```python
from build123d import *

# Parameters (mm, degrees)
SCHIZZO1_R                   = 15
SCHIZZO1_R_2                 = 5
ESTRUSIONE_ESTRUSIONE3_DEPTH = 10
ESTRUSIONE_ESTRUSIONE4_DEPTH = 6
RACCORDO1_R                  = 2
RACCORDO2_R                  = 4


with BuildPart() as part:
    # Schizzo1 → Estrusione-Estrusione3 (new, symmetric)
    with BuildSketch(Plane(origin=(0, 0, 0), x_dir=(1, 0, 0), z_dir=(0, 1, 0))):
        with BuildLine():
            Line((-9.947570822, 81.022660617), (-15.953490717, 22.602190996))
            ThreePointArc((-15.953490717, 22.602190996), (-19.887097519, 10.546739253), (-28.450004541, 1.193461616))
            Line((-28.450004541, 1.193461616), (-75.064098517, -31.841096257))
            ThreePointArc((-75.064098517, -31.841096257), (-77.965975808, -44.958742299), (-65.193896965, -49.126179346))
            Line((-65.193896965, -49.126179346), (-11.597326225, -25.117223738))
            ThreePointArc((-11.597326225, -25.117223738), (0.80980464, -22.496101285), (13.191434192, -25.235157478))
            Line((13.191434192, -25.235157478), (65.107247501, -49.0868681))
            ThreePointArc((65.107247501, -49.0868681), (77.918400858, -45.041144531), (75.141467788, -31.896481271))
            Line((75.141467788, -31.896481271), (27.550816942, 2.515032742))
            ThreePointArc((27.550816942, 2.515032742), (19.077292879, 11.949362033), (15.258570349, 24.041695862))
            Line((15.258570349, 24.041695862), (9.956851016, 80.927964356))
            ThreePointArc((9.956851016, 80.927964356), (0.047574951, 89.999886831), (-9.947570822, 81.022660617))
        make_face()
        with Locations(Location((0, 0, 0), (0, 0, 270))):
            Circle(SCHIZZO1_R, mode=Mode.SUBTRACT)
        with Locations(Location((0, 80, 0), (0, 0, 270))):
            Circle(SCHIZZO1_R_2, mode=Mode.SUBTRACT)
        with Locations(Location((69.282032303, -40, 0), (0, 0, 270))):
            Circle(SCHIZZO1_R_2, mode=Mode.SUBTRACT)
        with Locations(Location((-69.282032303, -40, 0), (0, 0, 270))):
            Circle(SCHIZZO1_R_2, mode=Mode.SUBTRACT)
        with BuildLine():
            Line((-5.859435485, 71.896481271), (-11.573917762, 16.31086839))
            ThreePointArc((-11.573917762, 16.31086839), (0, 20), (11.573917762, 16.31086839))
            Line((11.573917762, 16.31086839), (5.859435485, 71.896481271))
            ThreePointArc((5.859435485, 71.896481271), (0, 70), (-5.859435485, 71.896481271))
        make_face(mode=Mode.SUBTRACT)
        with BuildLine():
            Line((65.193896965, -30.873820654), (19.912585265, 1.867872608))
            ThreePointArc((19.912585265, 1.867872608), (17.320508076, -10), (8.338667503, -18.178740998))
            Line((8.338667503, -18.178740998), (59.334461481, -41.022660617))
            ThreePointArc((59.334461481, -41.022660617), (60.621778265, -35), (65.193896965, -30.873820654))
        make_face(mode=Mode.SUBTRACT)
        with BuildLine():
            Line((-59.334461481, -41.022660617), (-8.338667503, -18.178740998))
            ThreePointArc((-8.338667503, -18.178740998), (-17.320508076, -10), (-19.912585265, 1.867872608))
            Line((-19.912585265, 1.867872608), (-65.193896965, -30.873820654))
            ThreePointArc((-65.193896965, -30.873820654), (-60.621778265, -35), (-59.334461481, -41.022660617))
        make_face(mode=Mode.SUBTRACT)
    extrude(amount=ESTRUSIONE_ESTRUSIONE3_DEPTH, both=True)

    # Schizzo1_2 → Estrusione-Estrusione4 (add, symmetric)
    with BuildSketch(Plane(origin=(0, 0, 0), x_dir=(1, 0, 0), z_dir=(0, 1, 0))):
        with BuildLine():
            ThreePointArc((-19.912585265, 1.867872608), (-17.320508076, -10), (-8.338667503, -18.178740998))
            Line((-8.338667503, -18.178740998), (-59.334461481, -41.022660617))
            ThreePointArc((-59.334461481, -41.022660617), (-60.621778265, -35), (-65.193896965, -30.873820654))
            Line((-65.193896965, -30.873820654), (-19.912585265, 1.867872608))
        make_face()
        with BuildLine():
            ThreePointArc((11.573917762, 16.31086839), (0, 20), (-11.573917762, 16.31086839))
            Line((-11.573917762, 16.31086839), (-5.859435485, 71.896481271))
            ThreePointArc((-5.859435485, 71.896481271), (0, 70), (5.859435485, 71.896481271))
            Line((5.859435485, 71.896481271), (11.573917762, 16.31086839))
        make_face()
        with BuildLine():
            ThreePointArc((65.193896965, -30.873820654), (60.621778265, -35), (59.334461481, -41.022660617))
            Line((59.334461481, -41.022660617), (8.338667503, -18.178740998))
            ThreePointArc((8.338667503, -18.178740998), (17.320508076, -10), (19.912585265, 1.867872608))
            Line((19.912585265, 1.867872608), (65.193896965, -30.873820654))
        make_face()
    extrude(amount=ESTRUSIONE_ESTRUSIONE4_DEPTH, both=True)

    # Raccordo1
    raccordo1_edges = [part.edges().sort_by_distance(p)[0] for p in [
        (-59.334461481, -8, 41.022660617),
        (5.859435485, -8, -71.896481271),
        (-5.859435485, -8, -71.896481271),
        (59.334461481, -8, 41.022660617),
        (65.193896965, -8, 30.873820654),
        (5.859435485, 8, -71.896481271),
        (-5.859435485, 8, -71.896481271),
        (59.334461481, 8, 41.022660617),
        (65.193896965, 8, 30.873820654),
        (-65.193896965, 8, 30.873820654),
        (-59.334461481, 8, 41.022660617),
        (-65.193896965, -8, 30.873820654),
    ]]
    fillet(raccordo1_edges, radius=RACCORDO1_R)

    # Raccordo2
    raccordo2_edges = [part.edges().sort_by_distance(p)[0] for p in [
        (11.573917762, -8, -16.31086839),
        (-11.573917762, -8, -16.31086839),
        (8.338667503, -8, 18.178740998),
        (19.912585265, -8, -1.867872608),
        (-11.573917762, 8, -16.31086839),
        (11.573917762, 8, -16.31086839),
        (19.912585265, 8, -1.867872608),
        (8.338667503, 8, 18.178740998),
        (-8.338667503, 8, 18.178740998),
        (-19.912585265, 8, -1.867872608),
        (-19.912585265, -8, -1.867872608),
        (-8.338667503, -8, 18.178740998),
    ]]
    fillet(raccordo2_edges, radius=RACCORDO2_R)


solid = part.part
```
Source: CAD feature listing. Evaluate the final solid. Frame: model axes, mm. A direction names the side the tool comes from. Round coordinates to 2 decimals unless told otherwise and drop trailing zeros. Loops run counter-clockwise (first coordinate to the right, second up) from the corner with the lowest first, then second, coordinate; pieces in that order, holes last. Notation, with made-up numbers: M 55.25,14.5 L 82.25,14.5 A25 ccw 82.25,45.5 Z; hole C -31.75,56.25 d4. An arc over 180 degrees is marked long. Use a Markdown table: item, result. Add a question column.
1. Cut plane D-D, the plane y = 2.5. Output: boundary loops of the cut face in (x, z).
2. Cut plane B-B, the plane z = -10. Output: boundary loops of the cut face in (x, y).
3. Contact query for flat-ended pins moving along their axis: pin 1 (6 mm diameter, centred on x = -31.5, y = -4, fed in from +Z); pin 2 (11.5 mm diameter, centred on x = 69.28, z = 40, fed in from -Y); pin 3 (11.5 mm diameter, centred on x = 29.5, z = 16.5, fed in from -Y); pin 4 (5 mm diameter, centred on x = 22, y = 8, fed in from -Z). Output: stop coordinate, or through.
4. Cut plane C-C, the plane x = -33. Output: boundary loops of the cut face in (y, z), and give its area (3 significant figures).
5. Cut plane A-A, the plane x = 0. Output: boundary loops of the cut face in (y, z), and give its area (3 significant figures).
6. Set-up query: faces 4 (the cylindrical face through (0, 8, -70)), 5 (the flat face through (38, -6, 21)), 6 (the flat face through (38.8, 0.1, 37)). Return all of +Z, -Z, +X, -X, +Y, -Y with unobstructed straight access to the full face (end or side cutting, diameter ignored); none if empty.
7. Ray query, line 1 along X through (y, z) = (8, 27); line 2 along X through (y, z) = (8, 36.5); line 3 along X through (y, z) = (-2, 40). Return the intervals inside material, ascending. Write a range as [from, to].
8. Pull-direction query (X, two-part tool) for faces 1 (the cylindrical face through (-60.647, 7.972, 34.957)), 2 (the flat face through (51.68, 0.14, 14.93)), 3 (the cylindrical face through (-19.8, 0.1, -10.7)); classes: +X half, -X half, draft (parallel to the pull), parting line (faces both ways), or undercut.
Solution:
| question | item | result |
|---|---|---|
| 1 | outline | M -75.06,31.84 L -28.45,-1.19 A30 cw -15.95,-22.6 L -9.95,-81.02 A10 ccw 9.96,-80.93 L 15.26,-24.04 A30 cw 27.55,-2.52 L 75.14,31.9 A10 ccw 65.11,49.09 L 13.19,25.24 A30 cw -11.6,25.12 L -65.19,49.13 A10 ccw Z; hole C -69.28,40 d10; hole C 0,0 d30; hole C 0,-80 d10; hole C 69.28,40 d10 |
| 2 | outline | M -20.21,-10 L -11.18,-10 L -11.18,10 L -20.21,10 Z; M 11.18,-10 L 20.29,-10 L 20.29,10 L 11.18,10 Z |
| 3 | pin 1 | stops at z = 35.38 |
| 3 | pin 2 | stops at y = -10 |
| 3 | pin 3 | stops at y = -6 |
| 3 | pin 4 | stops at z = -11.23 |
| 4 | outline | M -10,2.03 L 10,2.03 L 10,7.6 L 6,7.6 L 6,29.23 L 10,29.23 L 10,34.7 L -10,34.7 L -10,29.23 L -6,29.23 L -6,7.6 L -10,7.6 Z |
| 4 | area | 480 mm2 |
| 5 | outline | M -10,-90 L 10,-90 L 10,-85 L -10,-85 Z; M -10,-75 L 10,-75 L 10,-70 L 6,-70 L 6,-20 L 10,-20 L 10,-15 L -10,-15 L -10,-20 L -6,-20 L -6,-70 L -10,-70 Z; M -10,15 L 10,15 L 10,22.5 L -10,22.5 Z |
| 5 | area | 1,050 mm2 |
| 6 | face 4 | +Y |
| 6 | face 5 | -Y |
| 6 | face 6 | +Z, +Y, -Y |
| 7 | line 1 | x = [-68.23, -59.84], [-28.03, -15.8], [17.03, 28.03], [59.84, 68.37] |
| 7 | line 2 | x = [-78.65, -72.85], [-65.71, -59.91], [-49.24, -37.01], [37.71, 49.24], [59.91, 65.71], [72.85, 78.65] |
| 7 | line 3 | x = [-79.28, -74.28], [-64.28, -44.82], [45.33, 64.28], [74.28, 79.28] |
| 8 | face 1 | undercut |
| 8 | face 2 | +X half |
| 8 | face 3 | -X half |
